Here's how the part is built. I have some questions about the finished solid (model axes, mm). Round coordinates to 2 decimals unless told otherwise and drop trailing zeros. Loops run counter-clockwise (first coordinate to the right, second up) from the corner with the lowest first, then second, coordinate; pieces in that order, holes last. Notation, with made-up numbers: M 25,32.5 L 58,32.5 A37 ccw 58,70.5 Z; hole C 31.25,47.25 d8. An arc over 180 degrees is marked long. Answer as a JSON object with one key per item and string values.
from build123d import *

# Parameters (mm, degrees)
SKETCH1_R            = 38.1
EXTRUDE2_DEPTH       = 12.7
SKETCH5_R            = 21.59
EXTRUDE3_DEPTH       = 56.358016583
EXTRUDE4_DEPTH       = 56.358016583
EXTRUDE4_DEPTH_BACK  = 56.358016583
EXTRUDE5_DEPTH       = 56.358016583
EXTRUDE5_DEPTH_BACK  = 56.358016583
M6_CLEARANCE_HOLE1_D = 6.4


with BuildPart() as part:
    # Sketch1 → Extrude2 (new body)
    with BuildSketch(Plane(origin=(0, 0, 0), x_dir=(1, 0, 0), z_dir=(0, 1, 0))):
        with Locations(Location((0, 0, 0), (0, 0, 270))):
            Circle(SKETCH1_R)
    extrude(amount=-EXTRUDE2_DEPTH)

    # Sketch5 → Extrude3 (cut, through all)
    with BuildSketch(Plane(origin=(0, 0, 0), x_dir=(1, 0, 0), z_dir=(0, 1, 0))):
        with Locations(Location((0, 0, 0), (0, 0, 270))):
            Circle(SKETCH5_R)
    extrude(amount=-EXTRUDE3_DEPTH, mode=Mode.SUBTRACT)

    # Sketch6 → Extrude4 (cut, two sides: drawn at the far end of the back side and taken through both)
    with BuildSketch(Plane(origin=(0, 0, 0), x_dir=(1, 0, 0), z_dir=(0, 1, 0)).offset(-EXTRUDE4_DEPTH_BACK)):
        Polygon((-213.093459479, 32.268567529), (-20.257086404, 32.268567529), (20.257086404, 32.268567529), (213.093459479, 32.268567529), (213.093459479, 417.941313679), (-213.093459479, 417.941313679), align=None)
    extrude(amount=EXTRUDE4_DEPTH + EXTRUDE4_DEPTH_BACK, mode=Mode.SUBTRACT)

    # Sketch7 → Extrude5 (cut, two sides: drawn at the far end of the back side and taken through both)
    with BuildSketch(Plane(origin=(0, 0, 0), x_dir=(1, 0, 0), z_dir=(0, 1, 0)).offset(-EXTRUDE5_DEPTH_BACK)):
        Polygon((-204.275376653, -32.268567529), (-20.257086404, -32.268567529), (20.257086404, -32.268567529), (204.275376653, -32.268567529), (204.275376653, -400.305148026), (-204.275376653, -400.305148026), align=None)
    extrude(amount=EXTRUDE5_DEPTH + EXTRUDE5_DEPTH_BACK, mode=Mode.SUBTRACT)

    # M6 Clearance Hole1 (through all)
    with Locations(Plane(origin=(8.636, -6.35, -32.268567529), x_dir=(-1, 0, 0), z_dir=(0, 0, -1))):
        with Locations((0, 0), (17.272, 0)):
            Hole(M6_CLEARANCE_HOLE1_D / 2)


solid = part.part
Item 1: Please list where these lines run through material, in increasing order: probe 1 along X at (y, z) = (-6.35, 25); probe 2 along X at (y, z) = (-6.35, -28.5); probe 3 along Z at (x, y) = (-4, -6.5). Write a range as from..to.
Resolved:
{"probe 1": "-28.75..-11.84, -5.44..5.44, 11.84..28.75", "probe 2": "-25.29..-11.84, -5.44..5.44, 11.84..25.29", "probe 3": "-32.27..-21.22, 21.22..32.27"}
Item 2: I want a section at C-C, the plane y = -11.25. Please give me the cut outline in (x, z), then the cut area to 3 significant figures.
Resolved:
{"outline": "M -20.26,-32.27 L 20.26,-32.27 A38.1 ccw 20.26,32.27 L -20.26,32.27 A38.1 ccw Z; hole C 0,0 d43.18", "area": "2,780 mm²"}
Item 3: I'm going to push flat-ended pins straight in: pin 1 Ø8 at (x, z) = (-22.5, -13) entering from +Y; pin 2 Ø4 at (x, y) = (-23, -8) entering from -Z; pin 3 Ø1 at (y, z) = (-4.5, -21) entering from +X; pin 4 Ø2 at (y, z) = (-9, -22.5) entering from +X. Where does each tip first touch, or does it pass through?
Resolved:
{"pin 1": "y = 0", "pin 2": "z = -31.79", "pin 3": "x = 32.11", "pin 4": "x = 31.45"}
Item 4: I want a section at B-B, the plane x = 3. Please give me the cut outline in (y, z), then the cut area to 3 significant figures.
Resolved:
{"outline": "M -12.7,-32.27 L 0,-32.27 L 0,-21.38 L -12.7,-21.38 Z; M -12.7,21.38 L 0,21.38 L 0,32.27 L -12.7,32.27 Z", "area": "277 mm²"}
Item 5: I want a section at D-D, the plane y = -6.35. Please give me the cut outline in (x, z).
Resolved:
{"outline": "M -20.26,-32.27 L -11.84,-32.27 L -11.84,-18.06 A21.59 cw -11.84,18.06 L -11.84,32.27 L -20.26,32.27 A38.1 ccw Z; M -5.44,-32.27 L 5.44,-32.27 L 5.44,-20.89 A21.59 cw -5.44,-20.89 Z; M -5.44,20.89 A21.59 cw 5.44,20.89 L 5.44,32.27 L -5.44,32.27 Z; M 11.84,-32.27 L 20.26,-32.27 A38.1 ccw 20.26,32.27 L 11.84,32.27 L 11.84,18.06 A21.59 cw 11.84,-18.06 Z"}
Item 6: I want a section at A-A, the plane z = 0. Please give me the cut outline in (x, y), then the cut area to 3 significant figures.
Resolved:
{"outline": "M -38.1,-12.7 L -21.59,-12.7 L -21.59,0 L -38.1,0 Z; M 21.59,-12.7 L 38.1,-12.7 L 38.1,0 L 21.59,0 Z", "area": "419 mm²"}
Item 7: If we mould it in two halves opening along X, with no side actions, what happens to faces 1 (the face through (1, -12.7, -22)), 2 (the face through (-11.833, -6.209, -26.616)), 3 (the face through (-38.096, -6.261, -0.539))? For each: pulls with the +X half, pulls with the -X half, needs draft (parallel to the pull), parting line crosses it, or undercut.
Resolved:
{"face 1": "needs draft", "face 2": "undercut", "face 3": "pulls with the -X half"}
